The model under review builds one solid part; all positions refer to its coordinate system, in mm. Round coordinates to 2 decimals unless told otherwise and drop trailing zeros. Loops run counter-clockwise (first coordinate to the right, second up) from the corner with the lowest first, then second, coordinate; pieces in that order, holes last. Notation, with made-up numbers: M -40,46 L -23,46 A24 ccw -23,67 Z; hole C 70.25,86 d6. An arc over 180 degrees is marked long. Return JSON: item names as keys, results as strings. Group by question number.
Q1. To check wall thickness, follow line 1 along Y through (x, z) = (-2, 21.5); line 2 along Y through (x, z) = (0.1, 21); line 3 along X through (y, z) = (-2.3, 9). State the ranges of each line that lie inside material, in increasing order.
Q2. Consider section A-A (z = 23.5). State the section outline as (x, y) points, and give its area (3 significant figures).
Q3. Clearance check with flat-ended pins moving along their axes: pin 1 Ø0.6 at (x, y) = (-2.5, -0.5) entering from -Z; pin 2 Ø1.5 at (y, z) = (-1.5, 7.5) entering from +X; pin 3 Ø2 at (y, z) = (0, 3) entering from -X; pin 4 Ø3 at (y, z) = (0.5, 16.5) entering from +X. State where each tip first meets the part, or that it passes through.
from build123d import *

# Parameters (mm, degrees)
SKETCH1_R           = 3
BOSS_EXTRUDE1_DEPTH = 35
SKETCH2_W           = 10
SKETCH2_H           = 6
CUT_EXTRUDE1_DEPTH  = 1
CHAMFER1_SIZE       = 0.2
SKETCH3_R           = 0.3
CUT_EXTRUDE2_DEPTH  = 0.4
CUT_EXTRUDE2_DRAFT  = -15


with BuildPart() as part:
    # Sketch1 → Boss-Extrude1 (new body)
    with BuildSketch(Plane.XY):
        Circle(SKETCH1_R)
    extrude(amount=BOSS_EXTRUDE1_DEPTH)

    # Sketch2 → Cut-Extrude1 (cut)
    with BuildSketch(Plane.ZY.offset(3)):
        with Locations((5, 0)):
            Rectangle(SKETCH2_W, SKETCH2_H)
    extrude(amount=-CUT_EXTRUDE1_DEPTH, mode=Mode.SUBTRACT)

    # Chamfer1
    chamfer1_edges = [part.edges().sort_by_distance(p)[0] for p in [
        (1.224744871, 2.738612788, 0),
        (-2, 0, 0),
        (-3, 0, 10),
        (-3, 0, 35),
    ]]
    chamfer(chamfer1_edges, length=CHAMFER1_SIZE)


with BuildPart() as cut_extrude2_tool:
    # Sketch3 → Cut-Extrude2 (with draft: the straight prism first)
    with BuildSketch(Plane(origin=(0, 0, 0), x_dir=(-1, 0, 0), z_dir=(0, 0, -1))):
        Circle(SKETCH3_R)
    extrude(amount=-CUT_EXTRUDE2_DEPTH)
    # Cut-Extrude2: the draft: its side faces are tilted about the plane it starts from
    cut_extrude2_sides = [cut_extrude2_tool.faces().sort_by_distance(p)[0] for p in [
        (0.3, 0, 0.2),
    ]]
    draft(cut_extrude2_sides, Plane(origin=(0, 0, 0), x_dir=(-1, 0, 0), z_dir=(0, 0, -1)), CUT_EXTRUDE2_DRAFT)


with BuildPart() as part_1:
    add(part.part)

    # Cut-Extrude2: cut by cut_extrude2_tool
    add(cut_extrude2_tool.part, mode=Mode.SUBTRACT)


solid = part_1.part
Values:
{
 "1": {"line 1": "y = -2.24 to 2.24", "line 2": "y = -3 to 3", "line 3": "x = -1.93 to 1.93"},
 "2": {"outline": "C 0,0 d6", "area": "28.3 mm2"},
 "3": {"pin 1": "stops at z = 10", "pin 2": "stops at x = 2.9", "pin 3": "stops at x = -2", "pin 4": "stops at x = 3"}
}
